from build123d import *

# Parameters (mm, degrees)
F2_SIZE  = 0.5
F3_SIZE  = 0.5
F6_DEPTH = 3.9


with BuildPart() as f1:
    # F0 (on Front) → F1 (revolve)
    with BuildSketch(Plane.XZ):
        with BuildLine():
            add(Edge.make_bspline(
                [(1.5, 2.3895676483), (3.8476854245, 2.0883835805), (6.8060247503, 1.1954580218), (7.95, 0)],
                knots=[1.5645237171, 1.5645237171, 1.5645237171, 1.5645237171, 8.3338166527, 8.3338166527, 8.3338166527, 8.3338166527], degree=3))
            Line((7.95, 0), (10.65, 0))
            Line((10.65, 0), (10.65, 2.6))
            Line((10.65, 2.6), (6.05, 2.6))
            Line((6.05, 2.6), (6.05, 3))
            Line((6.05, 3), (4, 3))
            Line((4, 3), (4, 6.9))
            Line((4, 6.9), (0, 6.9))
            Line((0, 6.9), (0, 2.8895676483))
            Line((0, 2.8895676483), (1.5, 2.8895676483))
            Line((1.5, 2.8895676483), (1.5, 2.3895676483))
        make_face()
        with BuildLine():
            Line((0, 2.8895676483), (0, 2.5))
            add(Edge.make_bspline(
                [(0, 2.5), (0.4474217695, 2.4971784695), (0.9574013029, 2.4591775207), (1.5, 2.3895676483)],
                knots=[0, 0, 0, 0, 1.5645237171, 1.5645237171, 1.5645237171, 1.5645237171], degree=3))
            Line((1.5, 2.3895676483), (1.5, 2.8895676483))
            Line((1.5, 2.8895676483), (0, 2.8895676483))
        make_face()
    revolve(axis=Axis((0, 0, 3.45), (0, 0, -1)))

    # F2
    f2_edges = [f1.edges().sort_by_distance(p)[0] for p in [
        (-4, 0, 6.9),
    ]]
    chamfer(f2_edges, length=F2_SIZE)

    # F3
    f3_edges = [f1.edges().sort_by_distance(p)[0] for p in [
        (-10.65, 0, 0),
    ]]
    chamfer(f3_edges, length=F3_SIZE)

    # F5 (on offset) → F6 (cut)
    with BuildSketch(Plane.XY.offset(6.9)):
        with BuildLine():
            ThreePointArc((0.3, -2.9849623113), (2.2248595461, -2.0124611797), (3, 0))
            ThreePointArc((3, 0), (2.2248595461, 2.0124611797), (0.3, 2.9849623113))
            Line((0.3, 2.9849623113), (0.3, 0))
            Line((0.3, 0), (0.3, -2.9849623113))
        make_face()
        with BuildLine():
            Line((0.3, 0), (0.3, 2.9849623113))
            ThreePointArc((0.3, 2.9849623113), (0, 3), (-0.3, 2.9849623113))
            Line((-0.3, 2.9849623113), (-0.3, 0))
            Line((-0.3, 0), (0, 0))
            Line((0, 0), (0.3, 0))
        make_face()
        with BuildLine():
            ThreePointArc((-0.3, 2.9849623113), (0, 3), (0.3, 2.9849623113))
            Line((0.3, 2.9849623113), (0.3, 4.0277631488))
            Line((0.3, 4.0277631488), (-0.3, 4.0277631488))
            Line((-0.3, 4.0277631488), (-0.3, 2.9849623113))
        make_face()
        with BuildLine():
            Line((0.3, -4.2378189974), (0.3, -2.9849623113))
            ThreePointArc((0.3, -2.9849623113), (0, -3), (-0.3, -2.9849623113))
            Line((-0.3, -2.9849623113), (-0.3, -4.2378189974))
            Line((-0.3, -4.2378189974), (0.3, -4.2378189974))
        make_face()
        with BuildLine():
            ThreePointArc((-0.3, -2.9849623113), (0, -3), (0.3, -2.9849623113))
            Line((0.3, -2.9849623113), (0.3, 0))
            Line((0.3, 0), (0, 0))
            Line((0, 0), (-0.3, 0))
            Line((-0.3, 0), (-0.3, -2.9849623113))
        make_face()
        with BuildLine():
            Line((-0.3, 0), (-0.3, 2.9849623113))
            ThreePointArc((-0.3, 2.9849623113), (-3, 0), (-0.3, -2.9849623113))
            Line((-0.3, -2.9849623113), (-0.3, 0))
        make_face()
    extrude(amount=-F6_DEPTH, mode=Mode.SUBTRACT)


solid = f1.part
Work out the finished part from the listing and answer in its coordinate system (mm). A direction names the side the tool comes from. Give positions to 0.01 mm unless a question says otherwise; leave off trailing zeros. Answer in a Markdown table with one row per item. Add a question column.
Q1. Each of these flat-tipped pins is pushed along its axis until it touches: P1, Ø0.5, axis at y = 3.5, z = 4.5, coming from the +X side; P2, Ø5, axis at x = 8, y = 4, coming from the +Z side; P3, Ø1.5, axis at y = 5.5, z = 5.5, coming from the -X side; P4, Ø0.5, axis at y = 3.5, z = 4.5, coming from the -X side. Where does it stop, or does it pass through?
Q2. A tool of negligible diameter and unlimited length cuts with its end or side. For faces 4 (the cylindrical face through (-3, 0, 5)), 5 (the flat face through (0.3, -3.5, 5)), 6 (the cylindrical face through (-4, 0, 5)), from which of +Z, -Z, +X, -X, +Y, -Y can it reach the whole face along a straight path? Write none if from no direction.
Q3. Consider line 1 along Z through (x, y) = (6.5, 5.75); line 2 along X through (y, z) = (-1, 5.5); line 3 along Y through (x, z) = (1.5, 3.75). Determine where each line is inside the solid, lowest interval first.
Q4. Determine the mould class of faces 1 (the cylindrical face through (5.589, 2.317, 2.803)), 2 (the flat face through (-3, 1, 6.9)), 3 (the flat face through (-0.3, -3.5, 5)) for opening direction X: released by +X, released by -X, zero draft, split by the parting line, or undercut.
Solution:
| question | item | result |
|---|---|---|
| 1 | P1 | stops at x = 2.33 |
| 1 | P2 | stops at z = 2.6 |
| 1 | P3 | passes through |
| 1 | P4 | stops at x = -2.33 |
| 2 | face 4 | +Z |
| 2 | face 5 | +Z, +Y, -Y |
| 2 | face 6 | +Z, -X |
| 3 | line 1 | z = 0 to 2.6 |
| 3 | line 2 | x = -3.87 to -2.83, 2.83 to 3.87 |
| 3 | line 3 | y = -3.71 to -2.6, 2.6 to 3.71 |
| 4 | face 1 | split by the parting line |
| 4 | face 2 | zero draft |
| 4 | face 3 | undercut |
